CAD build for the part. Positions are in the model's coordinates, mm. A direction names the side the tool comes from. Round coordinates to 2 decimals unless told otherwise and drop trailing zeros. Order: outer loops, then holes, each group sorted by start corner. A loop starts at its lowest first (then second) coordinate and runs counter-clockwise, first axis right, second up. Notation, with made-up numbers: (77, -19) -> (115, -19) arc R21 ccw to (115, 18) -> close; hole circle Ø2 at (14.5, 59). An arc over 180 degrees is marked (long way). Return JSON: item names as keys, results as strings. Group by question number.
Q1. Which spindle directions (+Z, -Z, +X, -X, +Y, -Y) get a long thin tool onto all of the face, cutting with end or side? Do faces 1 (the flat face through (92, 52, 12.7)), 2 (the flat face through (19.05, 25, -1)). Say none if no direction does.
Q2. Cut at D-D (y = 3). Write the cut outline in (x, z), then the cut area to 3 significant figures.
Q3. Flat gauge pin, fed straight in: pin 1 (12 mm diameter, centred on x = 115, y = 21, fed in from +Z). Where does the tip first touch, or does it go through?
Q4. Cut at B-B (y = 40). Write the cut outline in (x, z), then the cut area to 3 significant figures.
Q5. Probe line 1 along Y through (x, z) = (98, 9.5); line 2 along X through (y, z) = (12.5, 10); line 3 along Z through (x, y) = (59, 19.5). List the from-to ranges inside material, lowest first.
Q6. Cut at C-C (x = 153.5). Write the cut outline in (y, z).
Q7. Cut at A-A (z = 8). Write the cut outline in (x, y), then the cut area to 3 significant figures.
from build123d import *

# Parameters (mm, degrees)
F0_W     = 189.23
F0_H     = 55.88
F0_W_2   = 184.15
F0_H_2   = 50.8
F1_DEPTH = 12.7
F2_W     = 189.23
F2_H     = 55.88
F3_DEPTH = 6.35
F4_W     = 19.05
F4_H     = 50.8
F5_DEPTH = 3.81
F6_R     = 5.08


with BuildPart() as f1:
    # F0 (on Top) → F1 (new body)
    with BuildSketch(Plane.XY):
        with Locations((92.075, 25.4)):
            Rectangle(F0_W, F0_H)
        with Locations((92.075, 25.4)):
            Rectangle(F0_W_2, F0_H_2, mode=Mode.SUBTRACT)
    extrude(amount=F1_DEPTH)

    # F2 (on face) → F3 (join)
    with BuildSketch(Plane(origin=(0, 0, 0), x_dir=(1, 0, 0), z_dir=(0, 0, -1))):
        with Locations((92.075, -25.4)):
            Rectangle(F2_W, F2_H)
    extrude(amount=F3_DEPTH)

    # F4 (on face) → F5 (cut)
    with BuildSketch(Plane.XY):
        with Locations((9.525, 25.4)):
            Rectangle(F4_W, F4_H)
    extrude(amount=-F5_DEPTH, mode=Mode.SUBTRACT)

    # F6
    f6_edges = [f1.edges().sort_by_distance(p)[0] for p in [
        (101.6, 50.8, 0),
        (0, 50.8, 4.445),
        (184.15, 50.8, 6.35),
        (184.15, 25.4, 0),
        (184.15, 0, 6.35),
        (101.6, 0, 0),
        (0, 0, 4.445),
    ]]
    fillet(f6_edges, radius=F6_R)


solid = f1.part
Solution:
{
 "1": {"face 1": "+Z, +X, -X, +Y, -Y", "face 2": "+Z"},
 "2": {"outline": "(-2.54, -6.35) -> (186.69, -6.35) -> (186.69, 12.7) -> (183.7, 12.7) -> (183.7, 5.08) arc R4.63 cw to (179.07, 0.45) -> (19.05, 0.45) -> (19.05, -3.81) -> (0.45, -3.81) -> (0.45, 12.7) -> (-2.54, 12.7) -> close", "area": "1,280 mm²"},
 "3": {"pin 1": "stops at z = 0"},
 "4": {"outline": "(-2.54, -6.35) -> (186.69, -6.35) -> (186.69, 12.7) -> (184.15, 12.7) -> (184.15, 5.08) arc R5.08 cw to (179.07, 0) -> (19.05, 0) -> (19.05, -3.81) -> (0, -3.81) -> (0, 12.7) -> (-2.54, 12.7) -> close", "area": "1,200 mm²"},
 "5": {"line 1": "y = -2.54 to 0, 50.8 to 53.34", "line 2": "x = -2.54 to 0, 184.15 to 186.69", "line 3": "z = -6.35 to 0"},
 "6": {"outline": "(-2.54, -6.35) -> (53.34, -6.35) -> (53.34, 12.7) -> (50.8, 12.7) -> (50.8, 5.08) arc R5.08 cw to (45.72, 0) -> (5.08, 0) arc R5.08 cw to (0, 5.08) -> (0, 12.7) -> (-2.54, 12.7) -> close"},
 "7": {"outline": "(-2.54, -2.54) -> (186.69, -2.54) -> (186.69, 53.34) -> (-2.54, 53.34) -> close; hole (0, 5.08) arc R5.08 ccw to (5.08, 0) -> (179.07, 0) arc R5.08 ccw to (184.15, 5.08) -> (184.15, 45.72) arc R5.08 ccw to (179.07, 50.8) -> (5.08, 50.8) arc R5.08 ccw to (0, 45.72) -> close", "area": "1,240 mm²"}
}
